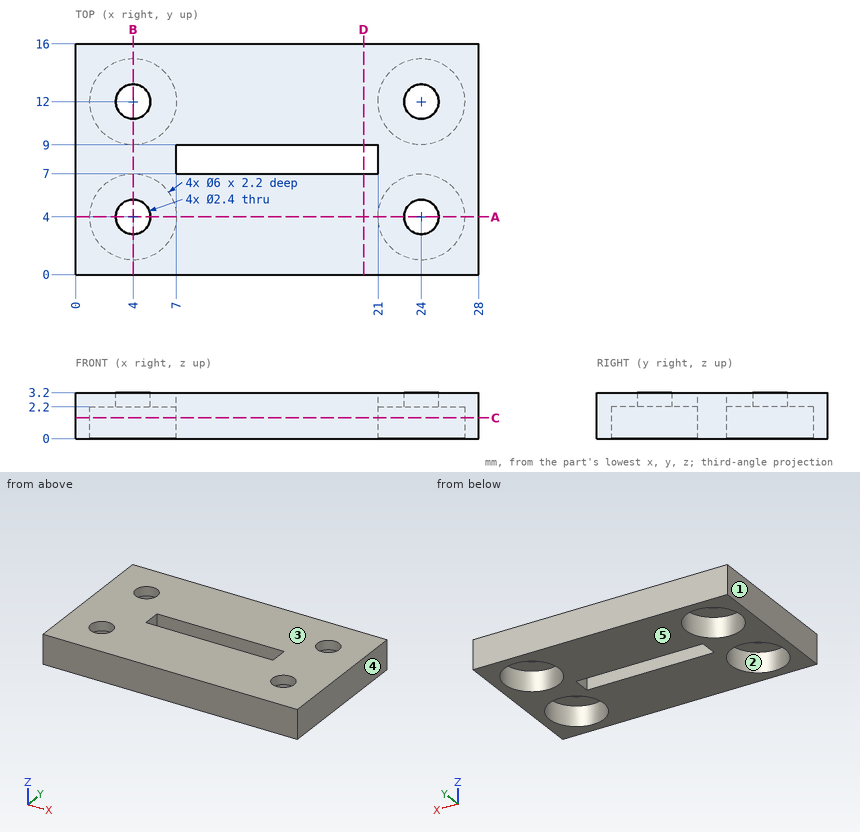
Source: three-view drawing plus pictorial views. Frame: mm from the lowest corner of the part. A direction names the side the tool comes from. Coordinates: 2 decimals unless noted, no trailing zeros. Loops run counter-clockwise (first coordinate to the right, second up) from the corner with the lowest first, then second, coordinate; pieces in that order, holes last. Notation, with made-up numbers: (51.25, 85.25) -> (76.25, 85.25) arc R25 cw to (76.25, 113.25) -> close; hole circle Ø10 at (7.5, -25.5). An arc over 180 degrees is marked (long way). Write each question's results on one line, items separated by ' | '. Start each with the question number.
Q1. Pin query (flat end, axial travel): pin 1 (3 mm diameter, centred on x = 4, y = 4, fed in from -Z). Return the tip coordinate at first contact, or that it passes through.
Q2. Ray query, line 1 (Y direction, x = 4, z = 0.9); line 2 (Y direction, x = 4, z = 2.8); line 3 (X direction, y = 12, z = 2.45). Return the intervals inside material, ascending. Write a range as from..to.
Q3. Section B-B, the plane x = 4. Return the cut outline in (y, z), plus the area to 3 significant figures.
Q4. Pull-direction query (Z, two-part tool) for the marked faces 3, 4 and 5; classes: released by +Z, released by -Z, zero draft, split by the parting line, or undercut.
Q5. Reachability of the marked faces 1 and 2 from +Z, -Z, +X, -X, +Y, -Y: full face, straight path, thin tool, end or side. Return the list, or none.
Q6. Section D-D, the plane x = 20. Return the cut outline in (y, z), plus the area to 3 significant figures.
Q7. Section C-C, the plane z = 1.45. Return the cut outline in (x, y), plus the area to 3 significant figures.
Q8. Section A-A, the plane y = 4. Return the cut outline in (x, z).
Found:
1) pin 1: z = 2.2
2) line 1: 0..1, 7..9, 15..16 | line 2: 0..2.8, 5.2..10.8, 13.2..16 | line 3: 0..2.8, 5.2..22.8, 25.2..28
3) outline: (0, 0) -> (1, 0) -> (1, 2.2) -> (2.8, 2.2) -> (2.8, 3.2) -> (0, 3.2) -> close; (5.2, 2.2) -> (7, 2.2) -> (7, 0) -> (9, 0) -> (9, 2.2) -> (10.8, 2.2) -> (10.8, 3.2) -> (5.2, 3.2) -> close; (13.2, 2.2) -> (15, 2.2) -> (15, 0) -> (16, 0) -> (16, 3.2) -> (13.2, 3.2) -> close | area: 20.0 mm2
4) face 3: released by +Z | face 4: zero draft | face 5: released by -Z
5) face 1: +Z, -Z, -X, +Y, -Y | face 2: -Z
6) outline: (0, 0) -> (7, 0) -> (7, 3.2) -> (0, 3.2) -> close; (9, 0) -> (16, 0) -> (16, 3.2) -> (9, 3.2) -> close | area: 44.8 mm2
7) outline: (0, 0) -> (28, 0) -> (28, 16) -> (0, 16) -> close; hole circle Ø6 at (4, 4); hole circle Ø6 at (4, 12); hole (7, 7) -> (21, 7) -> (21, 9) -> (7, 9) -> close; hole circle Ø6 at (24, 4); hole circle Ø6 at (24, 12) | area: 307 mm2
8) outline: (0, 0) -> (1, 0) -> (1, 2.2) -> (2.8, 2.2) -> (2.8, 3.2) -> (0, 3.2) -> close; (5.2, 2.2) -> (7, 2.2) -> (7, 0) -> (21, 0) -> (21, 2.2) -> (22.8, 2.2) -> (22.8, 3.2) -> (5.2, 3.2) -> close; (25.2, 2.2) -> (27, 2.2) -> (27, 0) -> (28, 0) -> (28, 3.2) -> (25.2, 3.2) -> close
